```python
from build123d import *

# Parameters (mm, degrees)
SKETCH1_W               = 34
SKETCH1_H               = 30
SKETCH1_R               = 5
BOSS_EXTRUDE1_DEPTH     = 30
CUT_EXTRUDE1_DEPTH      = 55.369108876
CUT_EXTRUDE1_DEPTH_BACK = 55.369108876
SKETCH2_R               = 2


with BuildPart() as part:
    # Sketch1 → Boss-Extrude1 (new body)
    with BuildSketch(Plane(origin=(0, 0, 0), x_dir=(1, 0, 0), z_dir=(0, 1, 0))):
        with Locations((17, -15)):
            Rectangle(SKETCH1_W, SKETCH1_H)
        with Locations(Location((17, -15, 0), (0, 0, 270))):
            Circle(SKETCH1_R, mode=Mode.SUBTRACT)
    extrude(amount=BOSS_EXTRUDE1_DEPTH)

    # Sketch2 → Cut-Extrude1 (cut, two sides: drawn at the far end of the back side and taken through both)
    with BuildSketch(Plane(origin=(0, 0, 0), x_dir=(-1, 0, 0), z_dir=(0, 0, -1)).offset(-CUT_EXTRUDE1_DEPTH_BACK)):
        with Locations((-29, 25)):
            Circle(SKETCH2_R)
        with Locations(Location((-5, 25, 0), (0, 0, 180))):
            Circle(SKETCH2_R)
        with Locations((-5, 5)):
            Circle(SKETCH2_R)
        with Locations(Location((-29, 5, 0), (0, 0, 180))):
            Circle(SKETCH2_R)
    extrude(amount=CUT_EXTRUDE1_DEPTH + CUT_EXTRUDE1_DEPTH_BACK, mode=Mode.SUBTRACT)


solid = part.part
```
Input: part model. Units: mm. Frame: model coordinates. Give positions to 0.01 mm unless a question says otherwise; leave off trailing zeros. Order: outer loops, then holes, each group sorted by start corner. A loop starts at its lowest first (then second) coordinate and runs counter-clockwise, first axis right, second up.
1. Cut plane C-C (z = 22.25). Return loops of the section in (x, y).
Computed:
outline: (0, 0) - (34, 0) - (34, 30) - (0, 30) - close; hole circle Ø4 at (5, 5); hole circle Ø4 at (5, 25); hole circle Ø4 at (29, 5); hole circle Ø4 at (29, 25)
2. Draft query along Y for faces 1 (the face through (17, 15, 30)), 2 (the face through (27.153, 24.234, 15.21)), 3 (the face through (13, 30, 11)). Return one class per face: released by +Y, released by -Y, zero draft, split by the parting line, or undercut.
Computed:
face 1: zero draft
face 2: undercut
face 3: released by +Y
3. Cut plane A-A (z = 15). Return loops of the section in (x, y).
Computed:
outline: (0, 0) - (12, 0) - (12, 30) - (0, 30) - close; (22, 0) - (34, 0) - (34, 30) - (22, 30) - close; hole circle Ø4 at (5, 5); hole circle Ø4 at (5, 25); hole circle Ø4 at (29, 5); hole circle Ø4 at (29, 25)
4. Line query: probe 1 along Y at (x, z) = (29, 15.5); probe 2 along X at (y, z) = (25.5, 3); probe 3 along X at (y, z) = (22.5, 14.75). Output: solid intervals per line, ascending.
Computed:
probe 1: y = 0 to 3, 7 to 23, 27 to 30
probe 2: x = 0 to 3.06, 6.94 to 27.06, 30.94 to 34
probe 3: x = 0 to 12.01, 21.99 to 34
5. Cut plane D-D (x = 29). Return loops of the section in (y, z).
Computed:
outline: (0, 0) - (3, 0) - (3, 30) - (0, 30) - close; (7, 0) - (23, 0) - (23, 30) - (7, 30) - close; (27, 0) - (30, 0) - (30, 30) - (27, 30) - close
6. Cut plane B-B (y = 5). Return loops of the section in (x, z).
Computed:
outline: (0, 0) - (3, 0) - (3, 30) - (0, 30) - close; (7, 0) - (27, 0) - (27, 30) - (7, 30) - close; (31, 0) - (34, 0) - (34, 30) - (31, 30) - close; hole circle Ø10 at (17, 15)
